Study the drawing (mm; zero at the part's minimum x, y, z) and answer. A direction names the side the tool comes from. Give positions to 0.01 mm unless a question says otherwise; leave off trailing zeros. Write each loop counter-clockwise with the first axis right and the second up, starting at its lowest first coordinate (ties: lowest second). Pieces come first, ordered by that corner, then holes. Notation, with made-up numbers: M 21.5,29 L 25.5,29 A35 ccw 25.5,68 Z; hole C 55,-28 d8. An arc over 180 degrees is marked long. Use a Markdown table: item, result. Add a question column.
Item 1: Consider probe 1 along Z at (x, y) = (19.05, 47.5); probe 2 along Y at (x, z) = (39, 47); probe 3 along Z at (x, y) = (49.5, 31.5). Determine where each line is inside the solid, lowest interval first. Write a range as [from, to].
Item 2: The mould has two halves that part along Z. Classify the marked faces 6, 7 and 8: pulls with the +Z half, pulls with the -Z half, needs draft (parallel to the pull), parting line crosses it, or undercut.
Item 3: For the marked faces 1, 2, 3, 4 and 5, determine the directions among +Z, -Z, +X, -X, +Y, -Y from which every point of the face is accessible in a straight line to the end or side of a thin tool.
Item 4: Given P1, Ø17, axis at x = 77.5, y = 38.5, coming from the -Z side; P2, Ø3, axis at y = 34.5, z = 3.5, coming from the -X side; P3, Ø2, axis at y = 38.5, z = 58, coming from the +X side (1 decimal); P4, Ø7.5, axis at x = 19.05, z = 57.15, coming from the -Y side, each flat-ended and moving along its own axis, determine where each tip first touches the part or whether it passes through.
Item 5: A cutting plane is placed at B-B on y = 38. Determine the outline of the cut face in (x, z), then the cut area to 3 significant figures.
Item 6: A cutting plane is placed at A-A on z = 57.15. Determine the outline of the cut face in (x, y), then the cut area to 3 significant figures.
Item 7: A cutting plane is placed at C-C on x = 19.05. Determine the outline of the cut face in (y, z).
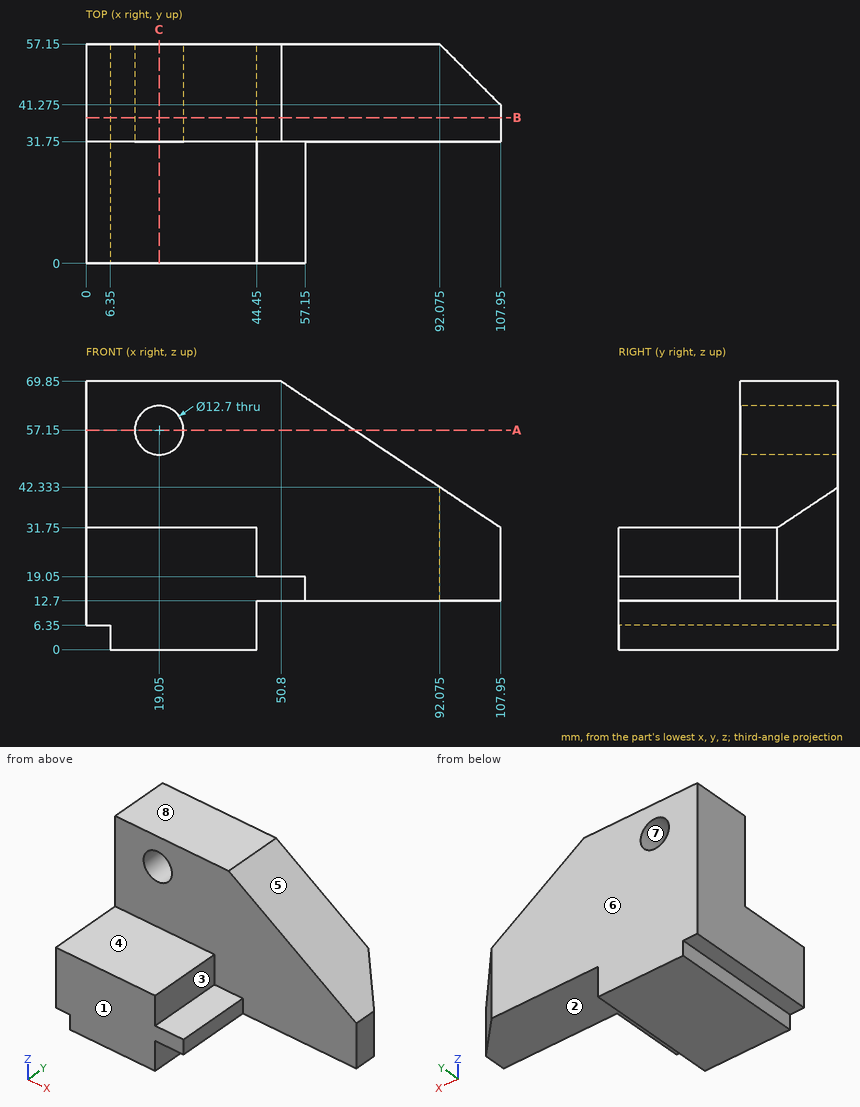
Filled in:
| question | item | result |
|---|---|---|
| 1 | probe 1 | [0, 50.8], [63.5, 69.85] |
| 1 | probe 2 | [31.75, 57.15] |
| 1 | probe 3 | [12.7, 19.05] |
| 2 | face 6 | needs draft |
| 2 | face 7 | undercut |
| 2 | face 8 | pulls with the +Z half |
| 3 | face 1 | +Z, -Z, +X, -X, -Y |
| 3 | face 2 | -Z, +X, +Y, -Y |
| 3 | face 3 | +Z, +X, -Y |
| 3 | face 4 | +Z, +X, -X, -Y |
| 3 | face 5 | +Z, +X, +Y, -Y |
| 4 | P1 | z = 12.7 |
| 4 | P2 | x = 6.35 |
| 4 | P3 | x = 70.1 |
| 4 | P4 | through |
| 5 | outline | M 0,6.35 L 6.35,6.35 L 6.35,0 L 44.45,0 L 44.45,12.7 L 107.95,12.7 L 107.95,31.75 L 50.8,69.85 L 0,69.85 Z; hole C 19.05,57.15 d12.7 |
| 5 | area | 5,480 mm² |
| 6 | outline | M 0,31.75 L 12.7,31.75 L 12.7,57.15 L 0,57.15 Z; M 25.4,31.75 L 69.85,31.75 L 69.85,57.15 L 25.4,57.15 Z |
| 6 | area | 1,450 mm² |
| 7 | outline | M 0,0 L 57.15,0 L 57.15,50.8 L 31.75,50.8 L 31.75,31.75 L 0,31.75 Z; M 31.75,63.5 L 57.15,63.5 L 57.15,69.85 L 31.75,69.85 Z |
